Source: CAD feature listing. Evaluate the final solid. Frame: model axes, mm. Face numbers are marked on the shaded views. A direction names the side the tool comes from. Give positions to 0.01 mm unless a question says otherwise; leave off trailing zeros. Order: outer loops, then holes, each group sorted by start corner. A loop starts at its lowest first (then second) coordinate and runs counter-clockwise, first axis right, second up.
1) Section C-C, the plane z = 15.5. Return loops of the section in (x, y).
2) First-contact query: P1, Ø1, axis at y = 42, z = 19, coming from the +X side; P2, Ø5, axis at y = 25, z = 6.5, coming from the +X side. Flat tips, straight axial feed; report the tip coordinate or a pass-through.
3) Draft query along Y for the marked faces 3, 4 and 5. Return one class per face: released by +Y, released by -Y, zero draft, split by the parting line, or undercut.
4) Section D-D, the plane x = 26. Return loops of the section in (y, z).
5) Section A-A, the plane z = 30. Return loops of the section in (x, y), plus the area to 3 significant figures.
6) Section B-B, the plane y = 21.5. Return loops of the section in (x, z), plus the area to 3 significant figures.
7) Material intervals for line 1 (X direction, y = 10, z = 11.5); line 2 (Z direction, x = 2, y = 9), sorted ascending.
8) Access query for the marked faces 1 and 2. Directions: +Z, -Z, +X, -X, +Y, -Y. A direction counts if a zero-diameter tool reaches every point of the face in a straight line with its end or side. Return the directions, or none.
Autodesk Inventor part; units mm, degrees
ref_plane "YZ Plane" through (0, 0, 0) normal (1, 0, 0) x (0, 1, 0)
ref_plane "XZ Plane" through (0, 0, 0) normal (0, 1, 0) x (-1, 0, 0)
ref_plane "XY Plane" through (0, 0, 0) normal (0, 0, 1) x (1, 0, 0)
sketch "Skizze1" plane through (0, 0, 0) normal (0, 0, 1) x (1, 0, 0)
  line L0 (0, 0) -> (0, 50)
  line L1 (0, 50) -> (48, 50)
  line L2 (53, 45) -> (53, 5)
  line L3 (48, 0) -> (0, 0)
  line L4 (12, 40) -> (42, 40) construction
  line L5 (12, 37.9) -> (42, 37.9)
  line L6 (42, 42.1) -> (12, 42.1)
  arc A0 (12, 42.1) -> (12, 37.9) centre (12, 40) ccw
  arc A1 (42, 37.9) -> (42, 42.1) centre (42, 40) ccw
  line L7 (12, 10) -> (42, 10) construction
  line L8 (12, 7.9) -> (42, 7.9)
  line L9 (42, 12.1) -> (12, 12.1)
  arc A2 (12, 12.1) -> (12, 7.9) centre (12, 10) ccw
  arc A3 (42, 7.9) -> (42, 12.1) centre (42, 10) ccw
  line L10 (48, 50) -> (53, 45)
  line L11 (53, 5) -> (48, 0)
  point P0 (53, 50)
  point P1 (53, 0)
  point P2 (27, 40)
  point P3 (27, 10)
  dimension "d0" = 50
  dimension "d1" = 53
  dimension "d2" = 30
  dimension "d3" = 4.2
  dimension "d4" = 10
  dimension "d5" = 11
  dimension "d6" = 4.2
  dimension "d7" = 10
  dimension "d8" = 11
  dimension "d9" = 5
  dimension "d10" = 5
  dimension "d11" = 5
  dimension "d12" = 5
extrude "Extrusion1" add sketch "Skizze1" along normal blind 3
sketch "Skizze2" plane through (0, 0, 0) normal (-1, 0, 0) x (0, 0, 1)
  line L0 (0, 50) -> (3, 50)
  line L1 (0, 50) -> (46, 50)
  line L2 (51, 45) -> (51, 5)
  line L3 (46, 0) -> (0, 0)
  line L4 (0, 0) -> (0, 50)
  line L5 (46, 50) -> (51, 45)
  line L6 (51, 5) -> (46, 0)
  circle A0 centre (30, 25) radius 11.05
  circle A1 centre (45.6319, 40.5) radius 1.75
  circle A2 centre (45.6319, 9.5) radius 1.75
  circle A3 centre (14.6319, 9.5) radius 1.75
  circle A4 centre (14.6319, 40.5) radius 1.75
  line L7 (30.1319, 50) -> (30.1319, 0) construction
  line L8 (51, 25) -> (0, 25) construction
  point P0 (51, 0)
  point P1 (51, 50)
  dimension "d15" = 51
  dimension "d16" = 5
  dimension "d17" = 5
  dimension "d18" = 5
  dimension "d19" = 5
  dimension "d20" = 22.1
  dimension "d21" = 3.5
  dimension "d22" = 21
  dimension "d23" = 3.5
  dimension "d24" = 3.5
  dimension "d25" = 3.5
  dimension "d26" = 31
  dimension "d27" = 31
  dimension "d28" = 31
  dimension "d29" = 31
  dimension "d30" = 15.5
  dimension "d31" = 15.5
  dimension "d32" = 15.5
  dimension "d33" = 15.5
extrude "Extrusion2" add sketch "Skizze2" against normal blind 3
sketch "Skizze3" plane through (0, 0, 0) normal (0, -1, 0) x (1, 0, 0)
  line L0 (3, 3) -> (48, 3)
  line L1 (8.8368, 3) -> (3, 8.8368)
  line L2 (8.8368, 3) -> (17.0913, 3) construction
  line L3 (3, 8.8368) -> (3, 26.8368)
  line L4 (3, 46) -> (3, 3)
  line L5 (3, 26.8368) -> (26.8368, 3)
  line L6 (42, 3) -> (12, 3)
  line L7 (26.8368, 3) -> (8.8368, 3)
  point P0 (0, 0)
  dimension "d36" = 135
  dimension "d37" = 18
  dimension "d38" = 45
extrude "Extrusion3" add sketch "Skizze3" against normal blind 3 contours L1 L3 L5 L0
sketch "Skizze4" plane through (0, 50, 0) normal (0, 1, 0) x (1, 0, 0)
  line L0 (42, -3) -> (12, -3)
  line L1 (3, -46) -> (3, -26.8368)
  line L2 (27, -3) -> (3, -26.8368)
  line L3 (8.8368, -3) -> (3, -8.8368)
  line L4 (3, -26.8368) -> (3, -8.8368)
  line L5 (3, -8.8368) -> (8.8368, -3)
  line L6 (8.8368, -3) -> (27, -3)
  point P0 (0, 0)
extrude "Extrusion4" add sketch "Skizze4" against normal blind 3
fillet "Rundung1" radius 2 2 edges at (0, 25, 0) (3, 25, 3)
properties part number "Motor mount NEMA 17" material "Stahl, unlegiert"
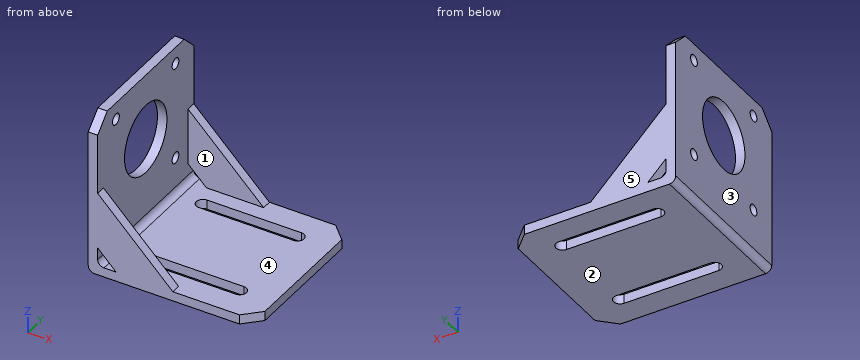
From the geometry:
1. outline: (0, 0) - (14.34, 0) - (14.34, 3) - (3, 3) - (3, 7.98) - (0, 7.98) - close; (0, 11.02) - (3, 11.02) - (3, 38.98) - (0, 38.98) - close; (0, 42.02) - (3, 42.02) - (3, 47) - (14.41, 47) - (14.41, 50) - (0, 50) - close
2. P1: stops at x = 3
2. P2: stops at x = 3.27
3. face 3: zero draft
3. face 4: undercut
3. face 5: released by +Y
4. outline: (0, 0) - (7.9, 0) - (7.9, 3) - (3, 3) - (3, 3.84) - (0, 3.84) - close; (12.1, 0) - (37.9, 0) - (37.9, 3) - (12.1, 3) - close; (42.1, 0) - (50, 0) - (50, 3.99) - (47, 3.99) - (47, 3) - (42.1, 3) - close
5. outline: (0, 0) - (3, 0) - (3, 13.95) - (0, 13.95) - close; (0, 36.05) - (3, 36.05) - (3, 50) - (0, 50) - close
5. area: 83.7 mm2
6. outline: (0, 2) arc R2 ccw to (2, 0) - (53, 0) - (53, 3) - (5, 3) arc R2 cw to (3, 5) - (3, 19.52) - (0, 19.52) - close; (0, 40.48) - (3, 40.48) - (3, 51) - (0, 51) - close
6. area: 240 mm2
7. line 1: x = 0 to 3
7. line 2: z = 0 to 12.95, 16.31 to 43.95, 47.31 to 51
8. face 1: +Z, +X
8. face 2: -Z, +X, -X, +Y, -Y
